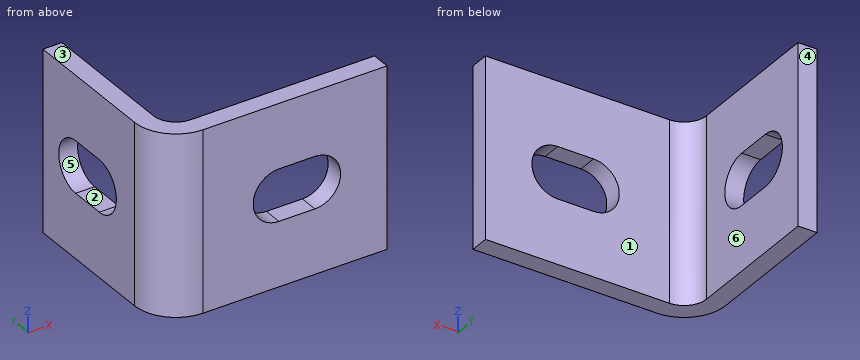
from build123d import *

# Parameters (mm, degrees)
BOSS_EXTRUDE1_DEPTH = 25.4
CUT_EXTRUDE1_DEPTH  = 47.218404224
CUT_EXTRUDE2_DEPTH  = 47.583385332


with BuildPart() as part:
    # Sketch2 → Boss-Extrude1 (new body)
    with BuildSketch(Plane.XY):
        with BuildLine():
            Line((0, 5.842), (0, 25.4))
            Line((0, 25.4), (2.667, 25.4))
            Line((2.667, 25.4), (2.667, 5.842))
            ThreePointArc((2.667, 5.842), (3.59693597, 3.59693597), (5.842, 2.667))
            Line((5.842, 2.667), (31.75, 2.667))
            Line((31.75, 2.667), (31.75, 0))
            Line((31.75, 0), (5.842, 0))
            ThreePointArc((5.842, 0), (1.711082184, 1.711082184), (0, 5.842))
        make_face()
    extrude(amount=BOSS_EXTRUDE1_DEPTH)

    # Sketch3 → Cut-Extrude1 (cut, through all)
    with BuildSketch(Plane(origin=(2.667, 0, 0), x_dir=(0, 0, -1), z_dir=(1, 0, 0))):
        with BuildLine():
            Line((-9.0678, 18.4023), (-9.0678, 13.3477))
            ThreePointArc((-9.0678, 13.3477), (-12.7, 9.7155), (-16.3322, 13.3477))
            Line((-16.3322, 13.3477), (-16.3322, 18.4023))
            ThreePointArc((-16.3322, 18.4023), (-12.7, 22.0345), (-9.0678, 18.4023))
        make_face()
    extrude(amount=-CUT_EXTRUDE1_DEPTH, mode=Mode.SUBTRACT)

    # Sketch4 → Cut-Extrude2 (cut, through all)
    with BuildSketch(Plane(origin=(0, 2.667, 0), x_dir=(1, 0, 0), z_dir=(0, 1, 0))):
        with BuildLine():
            Line((21.5773, -16.3322), (16.5227, -16.3322))
            ThreePointArc((16.5227, -16.3322), (12.8905, -12.7), (16.5227, -9.0678))
            Line((16.5227, -9.0678), (21.5773, -9.0678))
            ThreePointArc((21.5773, -9.0678), (25.2095, -12.7), (21.5773, -16.3322))
        make_face()
    extrude(amount=-CUT_EXTRUDE2_DEPTH, mode=Mode.SUBTRACT)


solid = part.part
Work out the finished part from the listing and answer in its coordinate system (mm). Face numbers are marked on the shaded views. A direction names the side the tool comes from. Round coordinates to 2 decimals unless told otherwise and drop trailing zeros. Order: outer loops, then holes, each group sorted by start corner. A loop starts at its lowest first (then second) coordinate and runs counter-clockwise, first axis right, second up. Notation, with made-up numbers: M -19,-3.5 L 14,-3.5 A10 cw 14,14.5 Z; hole C -30,26.25 d7. An arc over 180 degrees is marked long. One line per item, written item: value.
Q1. Find section D-D on z = 6.5. Write down the section's boundary in (x, y) (3 decimals), then the cut area to 3 significant figures.
Derived:
outline: M 0,5.842 A5.842 ccw 5.842,0 L 31.75,0 L 31.75,2.667 L 5.842,2.667 A3.175 cw 2.667,5.842 L 2.667,25.4 L 0,25.4 Z
area: 140 mm²
Q2. For the marked faces 4, 5 and 6, determine the directions among +Z, -Z, +X, -X, +Y, -Y from which every point of the face is accessible in a straight line to the end or side of a thin tool.
Derived:
face 4: +Z, -Z, +X, -X, +Y
face 5: +X, -X
face 6: +Z, -Z, +X, +Y
Q3. Flat-ended cylindrical pins translate along their axes: pin 1 (2 mm diameter, centred on y = 9.5, z = 13, fed in from +X); pin 2 (2 mm diameter, centred on x = 18, y = 1.5, fed in from -Z); pin 3 (3 mm diameter, centred on y = 3.5, z = 9, fed in from -X); pin 4 (6 mm diameter, centred on x = 27.5, z = 15, fed in from +Y). Find the tip coordinate at first contact, or state that the pin passes through.
Derived:
pin 1: x = 2.67
pin 2: z = 0
pin 3: x = 0.06
pin 4: y = 2.67
Q4. Determine the mould class of the marked faces 1, 2 and 3 for opening direction Z: released by +Z, released by -Z, zero draft, split by the parting line, or undercut.
Derived:
face 1: zero draft
face 2: undercut
face 3: released by +Z
Q5. Find section B-B on x = 18. Write down the section's boundary in (y, z).
Derived:
outline: M 0,0 L 2.67,0 L 2.67,9.07 L 0,9.07 Z; M 0,16.33 L 2.67,16.33 L 2.67,25.4 L 0,25.4 Z
Q6. Find section A-A on z = 12.7. Give the number of separate pieces and of enclosed holes in the cut face, then the cut area to 3 significant figures.
Derived:
separate pieces: 3
enclosed holes: 0
area: 74.4 mm²
Q7. Straight lines are drawn through the part: line 1 (Z direction, x = 20, y = 2.5); line 2 (Y direction, x = 28, z = 23). For each, find the intervals that lie inside material, in ascending order.
Derived:
line 1: 0 to 9.07, 16.33 to 25.4
line 2: 0 to 2.67
